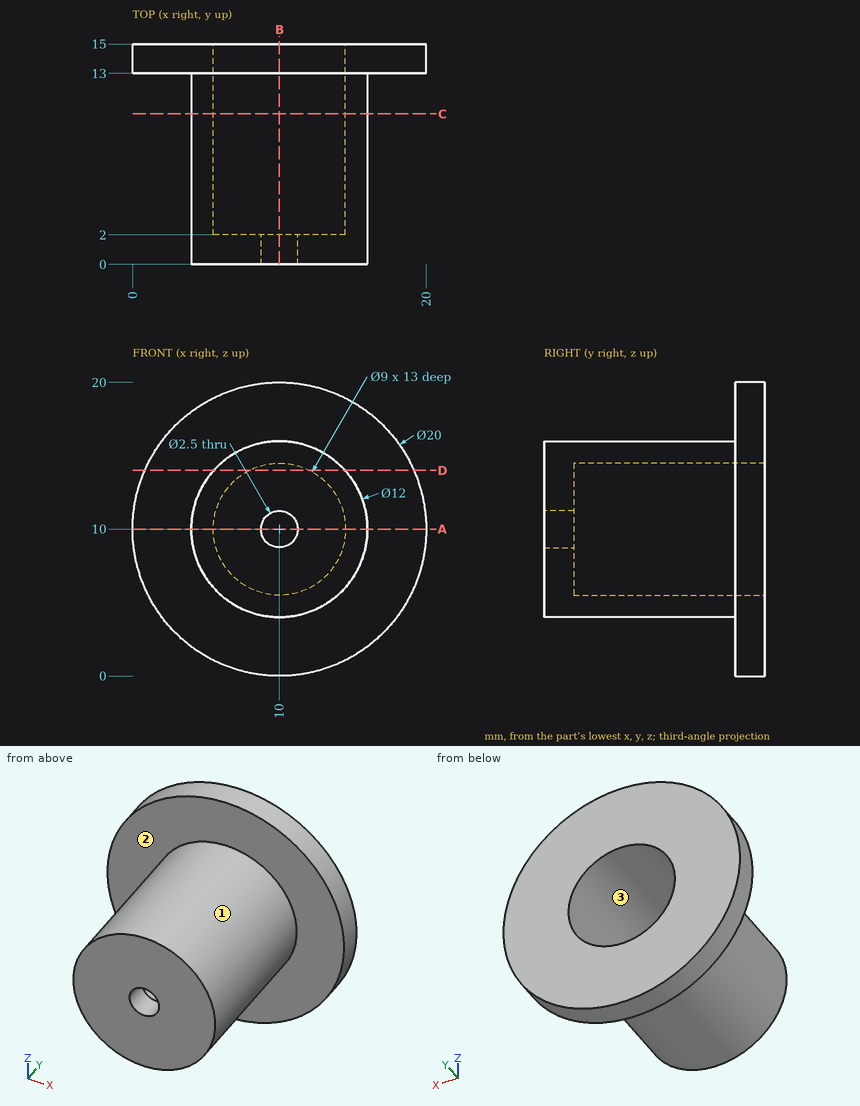
Answer from the drawing. Dimensions are ordinates in mm from the lowest x, y and z of the part. Coordinates: 2 decimals unless noted, no trailing zeros. Loops run counter-clockwise (first coordinate to the right, second up) from the corner with the lowest first, then second, coordinate; pieces in that order, holes last.
1) Flat-ended cylindrical pins translate along their axes: pin 1 (1 mm diameter, centred on x = 18, y = 8.5, fed in from +Z); pin 2 (4 mm diameter, centred on y = 9, z = 5, fed in from +X); pin 3 (1 mm diameter, centred on y = 11, z = 6, fed in from -X); pin 4 (4.5 mm diameter, centred on x = 9.5, z = 8.5, fed in from +Y). Find the tip coordinate at first contact, or state that the pin passes through.
Results:
pin 1: passes through
pin 2: stops at x = 15.2
pin 3: stops at x = 5.13
pin 4: stops at y = 2
2) Section A-A (z = 10) is taken. Give the vertices of the cut face in (x, y).
Results:
outline: (0, 13) - (4, 13) - (4, 0) - (8.75, 0) - (8.75, 2) - (5.5, 2) - (5.5, 15) - (0, 15) - close; (11.25, 0) - (16, 0) - (16, 13) - (20, 13) - (20, 15) - (14.5, 15) - (14.5, 2) - (11.25, 2) - close
3) Consider probe 1 along X at (y, z) = (11.75, 10); probe 2 along X at (y, z) = (0.9, 10); probe 3 along Z at (x, y) = (10.25, 14.25). Determine where each line is inside the solid, lowest interval first.
Results:
probe 1: x = 4 to 5.5, 14.5 to 16
probe 2: x = 4 to 8.75, 11.25 to 16
probe 3: z = 0 to 5.51, 14.49 to 20
4) Section C-C (y = 10.25) is taken. Give the vertices of the cut face in (x, z), plus the area to 3 significant figures.
Results:
outline: circle Ø12 at (10, 10); hole circle Ø9 at (10, 10)
area: 49.5 mm2
5) Section B-B (x = 10) is taken. Give the vertices of the cut face in (y, z).
Results:
outline: (0, 4) - (13, 4) - (13, 0) - (15, 0) - (15, 5.5) - (2, 5.5) - (2, 8.75) - (0, 8.75) - close; (0, 11.25) - (2, 11.25) - (2, 14.5) - (15, 14.5) - (15, 20) - (13, 20) - (13, 16) - (0, 16) - close
6) For a pull along Z with two mould halves and no side action, classify the marked faces 1, 2 and 3 as +Z half, -Z half, draft (parallel to the pull), parting line (faces both ways), or undercut.
Results:
face 1: parting line
face 2: draft
face 3: undercut
7) Section D-D (z = 14) is taken. Give the vertices of the cut face in (x, y).
Results:
outline: (0.83, 13) - (5.53, 13) - (5.53, 0) - (14.47, 0) - (14.47, 13) - (19.17, 13) - (19.17, 15) - (12.06, 15) - (12.06, 2) - (7.94, 2) - (7.94, 15) - (0.83, 15) - close
